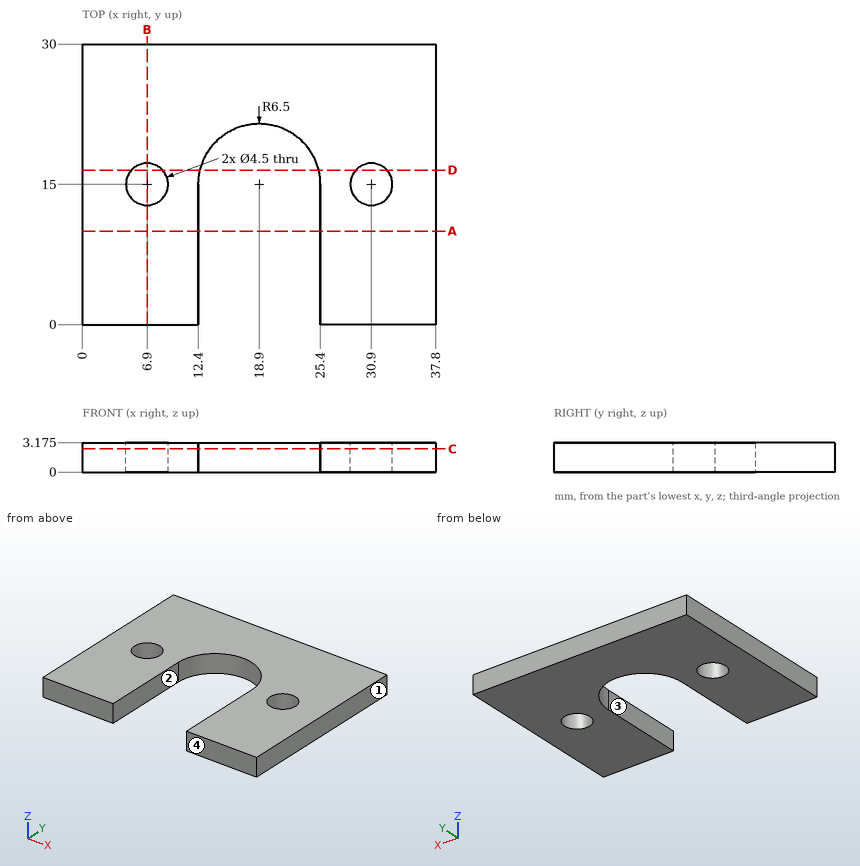
Can you work these out from the drawing? Everything is in mm from the part's minimum corner. Give positions to 0.01 mm unless a question says otherwise; leave off trailing zeros. Write each loop counter-clockwise with the first axis right and the second up, starting at its lowest first coordinate (ties: lowest second). Pieces come first, ordered by that corner, then holes. Notation, with made-up numbers: (50.5, 79) -> (55.5, 79) arc R18 cw to (55.5, 97) -> close; hole circle Ø11 at (-34.75, 12.25). An arc over 180 degrees is marked (long way). Write each question's results on one line, items separated by ' | '.
Item 1: Suppose I cut it at A-A on y = 10. Write out the boundary of the cut face in (x, z) (3 decimals).
Output:
outline: (0, 0) -> (12.4, 0) -> (12.4, 3.175) -> (0, 3.175) -> close; (25.4, 0) -> (37.8, 0) -> (37.8, 3.175) -> (25.4, 3.175) -> close
Item 2: For pin 1 Ø3.5 at (x, y) = (30.9, 15) entering from +Z, with a flat end and sliding along its axis, tell me the tip position at first contact or that it passes through.
Output:
pin 1: passes through
Item 3: Suppose I cut it at C-C on z = 2.5. Write out the boundary of the cut face in (x, y), plus the area to 3 significant figures.
Output:
outline: (0, 0) -> (12.4, 0) -> (12.4, 15) arc R6.5 cw to (25.4, 15) -> (25.4, 0) -> (37.8, 0) -> (37.8, 30) -> (0, 30) -> close; hole circle Ø4.5 at (6.9, 15); hole circle Ø4.5 at (30.9, 15) | area: 841 mm^2
Item 4: Suppose I cut it at D-D on y = 16.5. Write out the boundary of the cut face in (x, z) (3 decimals).
Output:
outline: (0, 0) -> (5.223, 0) -> (5.223, 3.175) -> (0, 3.175) -> close; (8.577, 0) -> (12.575, 0) -> (12.575, 3.175) -> (8.577, 3.175) -> close; (25.225, 0) -> (29.223, 0) -> (29.223, 3.175) -> (25.225, 3.175) -> close; (32.577, 0) -> (37.8, 0) -> (37.8, 3.175) -> (32.577, 3.175) -> close
Item 5: We'd pull the mould along X, two halves only. Please class the marked faces 1, 2, 3 and 4: pulls with the +X half, pulls with the -X half, needs draft (parallel to the pull), parting line crosses it, or undercut.
Output:
face 1: pulls with the +X half | face 2: undercut | face 3: undercut | face 4: needs draft
Item 6: If I drill on L1, parallel to X at y = 12, z = 1.3; L2, parallel to Y at x = 30.9, z = 2.3; L3, parallel to Y at x = 32.5, z = 2.4, over which ranges is the centre line in solid material (lowest first)?
Output:
L1: x = 0 to 12.4, 25.4 to 37.8 | L2: y = 0 to 12.75, 17.25 to 30 | L3: y = 0 to 13.42, 16.58 to 30
Item 7: Suppose I cut it at B-B on x = 6.9. Write out the boundary of the cut face in (y, z) (3 decimals), plus the area to 3 significant figures.
Output:
outline: (0, 0) -> (12.75, 0) -> (12.75, 3.175) -> (0, 3.175) -> close; (17.25, 0) -> (30, 0) -> (30, 3.175) -> (17.25, 3.175) -> close | area: 81.0 mm^2
